```python
from build123d import *

# Parameters (mm, degrees)
SKETCH_1_R          = 1.5
EXTRUDE_1_DEPTH     = 3
CUT_EXTRUDE_1_DEPTH = 3
FILLET_1_R          = 5


with BuildPart() as part:
    # 草图1 → 凸台-拉伸1 (new body)
    with BuildSketch(Plane.XY):
        with BuildLine():
            Line((-66.898598537, 2.653376251), (-33.898598537, 2.653376251))
            ThreePointArc((-33.898598537, 2.653376251), (1.101401463, -32.346623749), (36.101401463, 2.653376251))
            Line((36.101401463, 2.653376251), (69.101401463, 2.653376251))
            ThreePointArc((69.101401463, 2.653376251), (1.101401463, -65.346623749), (-66.898598537, 2.653376251))
        make_face()
        with Locations((-51.588074716, -3.346623749)):
            Circle(SKETCH_1_R, mode=Mode.SUBTRACT)
        with Locations((-4.898598537, -50.036099928)):
            Circle(SKETCH_1_R, mode=Mode.SUBTRACT)
        with Locations((7.101401463, -50.036099928)):
            Circle(SKETCH_1_R, mode=Mode.SUBTRACT)
        with Locations((53.790877642, -3.346623749)):
            Circle(SKETCH_1_R, mode=Mode.SUBTRACT)
    extrude(amount=EXTRUDE_1_DEPTH)

    # 草图2 → 切除-拉伸1 (cut)
    with BuildSketch(Plane.XY.offset(3)):
        with BuildLine():
            Line((10.319593038, -37.29690465), (15.041105796, -57.759243648))
            ThreePointArc((15.041105796, -57.759243648), (44.942021896, -41.187244183), (61.514021362, -11.286328082))
            Line((61.514021362, -11.286328082), (41.051682364, -6.564815324))
            ThreePointArc((41.051682364, -6.564815324), (30.092779491, -26.338001778), (10.319593038, -37.29690465))
        make_face()
        with BuildLine():
            Line((-8.116790112, -37.29690465), (-12.83830287, -57.759243648))
            ThreePointArc((-12.83830287, -57.759243648), (-42.739218971, -41.187244183), (-59.311218437, -11.286328082))
            Line((-59.311218437, -11.286328082), (-38.848879439, -6.564815324))
            ThreePointArc((-38.848879439, -6.564815324), (-27.889976566, -26.338001778), (-8.116790112, -37.29690465))
        make_face()
    extrude(amount=-CUT_EXTRUDE_1_DEPTH, mode=Mode.SUBTRACT)

    # 圆角1
    fillet_1_edges = [part.edges().sort_by_distance(p)[0] for p in [
        (-38.848879439, -6.564815324, 1.5),
        (-8.116790112, -37.29690465, 1.5),
        (-12.83830287, -57.759243648, 1.5),
        (-59.311218437, -11.286328082, 1.5),
        (10.319593038, -37.29690465, 1.5),
        (41.051682364, -6.564815324, 1.5),
        (61.514021362, -11.286328082, 1.5),
        (15.041105796, -57.759243648, 1.5),
    ]]
    fillet(fillet_1_edges, radius=FILLET_1_R)


solid = part.part
```
The listing builds one solid part. Answer for the finished solid, in the listing's coordinates (mm). A direction names the side the tool comes from. Coordinates: 2 decimals unless noted, no trailing zeros. Write each loop counter-clockwise with the first axis right and the second up, starting at its lowest first coordinate (ties: lowest second). Pieces come first, ordered by that corner, then holes.
Q1. Section B-B, the plane y = -47 is taken. Write down the section's boundary in (x, z).
Returned:
outline: (-45.36, 0) - (-36.03, 0) - (-36.03, 3) - (-45.36, 3) - close; (-10.36, 0) - (12.56, 0) - (12.56, 3) - (-10.36, 3) - close; (38.23, 0) - (47.56, 0) - (47.56, 3) - (38.23, 3) - close
Q2. The mould has two halves that part along Y. Classify faces 3 (the cylindrical face through (2.6, -65.33, 1.48)), 4 (the flat face through (-51, 2.653, 1)), 5 (the cylindrical face through (-28.072, -26.155, 1.521)): released by +Y, released by -Y, zero draft, split by the parting line, or undercut.
Returned:
face 3: released by -Y
face 4: released by +Y
face 5: undercut
Q3. Given P1, Ø2.5, axis at x = 53.79, y = -3.35, coming from the +Z side, flat-ended and moving along its own axis, determine where the tip first touches the part or whether it passes through.
Returned:
P1: passes through
Q4. Which of the six approach directions +Z, -Z, +X, -X, +Y, -Y give full straight-line access (tool end or side, diameter ignored) to faces 1 (the flat face through (51.12, -8.89, 1.52)), 2 (the cylindrical face through (0.33, -32.34, 1.48))?
Returned:
face 1: +Z, -Z
face 2: +Z, -Z, +Y
Q5. Section D-D, the plane y = -19.5 is taken. Write down the section's boundary in (x, z).
Returned:
outline: (-63.19, 0) - (-56.81, 0) - (-56.81, 3) - (-63.19, 3) - close; (-33.4, 0) - (-26, 0) - (-26, 3) - (-33.4, 3) - close; (28.2, 0) - (35.6, 0) - (35.6, 3) - (28.2, 3) - close; (59.01, 0) - (65.39, 0) - (65.39, 3) - (59.01, 3) - close
Q6. Section C-C, the plane z = 2.4 is taken. Write down the section's boundary in (x, y).
Returned:
outline: (-66.9, 2.65) arc R68 ccw to (69.1, 2.65) - (36.1, 2.65) arc R35 cw to (-33.9, 2.65) - close; hole (-57.86, -16.53) arc R62 ccw to (-18.08, -56.3) arc R5 ccw to (-11.66, -52.67) - (-9.18, -41.9) arc R5 ccw to (-12.4, -36.06) arc R41 cw to (-37.61, -10.85) arc R5 ccw to (-43.46, -7.63) - (-54.23, -10.11) arc R5 ccw to start; hole circle Ø3 at (-51.59, -3.35); hole circle Ø3 at (-4.9, -50.04); hole circle Ø3 at (7.1, -50.04); hole (11.38, -41.9) - (13.87, -52.67) arc R5 ccw to (20.29, -56.3) arc R62 ccw to (60.06, -16.53) arc R5 ccw to (56.43, -10.11) - (45.66, -7.63) arc R5 ccw to (39.81, -10.85) arc R41 cw to (14.61, -36.06) arc R5 ccw to start; hole circle Ø3 at (53.79, -3.35)
Q7. Section A-A, the plane x = 47 is taken. Write down the section's boundary in (y, z).
Returned:
outline: (-47.52, 0) - (-39.03, 0) - (-39.03, 3) - (-47.52, 3) - close; (-7.94, 0) - (2.65, 0) - (2.65, 3) - (-7.94, 3) - close
Q8. Find the intervals of material crossed by line 1 along X through (y, z) = (-18, 1.4); line 2 along X through (y, z) = (-53, 2.65); line 3 along X through (y, z) = (-18.5, 2.1), in increasing order.
Returned:
line 1: x = -63.69 to -57.36, -34.32 to -27.16, 29.36 to 36.52, 59.56 to 65.89
line 2: x = -37.97 to -26.22, -11.75 to 13.95, 28.43 to 40.17
line 3: x = -63.52 to -57.18, -34.02 to -26.78, 28.99 to 36.22, 59.38 to 65.73
